```python
from build123d import *

# Parameters (mm, degrees)
SKETCH_1_W      = 62.995
SKETCH_1_H      = 25
SKETCH_1_R      = 1.4
EXTRUDE_1_DEPTH = 2.5


with BuildPart() as part:
    # 草图1 → 凸台-拉伸1 (new body, symmetric)
    with BuildSketch(Plane(origin=(0, 0, 0), x_dir=(0, 0, -1), z_dir=(1, 0, 0))):
        with Locations((31.4975, 12.5)):
            Rectangle(SKETCH_1_W, SKETCH_1_H)
        with Locations((4.995, 4.5)):
            Circle(SKETCH_1_R, mode=Mode.SUBTRACT)
        with Locations((4.995, 20.5)):
            Circle(SKETCH_1_R, mode=Mode.SUBTRACT)
        with Locations((42.995, 12.5)):
            Circle(SKETCH_1_R, mode=Mode.SUBTRACT)
        with Locations((57.995, 12.5)):
            Circle(SKETCH_1_R, mode=Mode.SUBTRACT)
    extrude(amount=EXTRUDE_1_DEPTH, both=True)


solid = part.part
```
Read the model definition and answer for the solid it produces. Units are mm, in the model's axes. Give positions to 0.01 mm unless a question says otherwise; leave off trailing zeros. Loops run counter-clockwise (first coordinate to the right, second up) from the corner with the lowest first, then second, coordinate; pieces in that order, holes last.
Item 1: The part is cut by section C-C (x = -1). Write down the section's boundary in (y, z) (3 decimals).
Item 2: The part is cut by section D-D (y = 21.25). Write down the section's boundary in (x, z) (3 decimals), and give its area (3 significant figures).
Item 3: The part is cut by section A-A (y = 12.5). Write down the section's boundary in (x, z) (3 decimals).
Item 4: The part is cut by section B-B (y = 4.5). Write down the section's boundary in (x, z) (3 decimals), and give its area (3 significant figures).
Item 5: Find the intervals of material crossed by line 1 along Z through (x, y) = (-1, 13) (3 decimals); line 2 along Z through (x, y) = (-1.45, 12.75) (1 decimal); line 3 along Y through (x, z) = (0.1, -58.5), in increasing order.
Item 6: This flat-tipped pin is pushed along its axis until it touches: pin 1 Ø3 at (x, y) = (1, 4) entering from +Z. Where does it stop, or does it pass through?
Item 7: The mould has two halves that part along Y. Classify faces 1 (the flat face through (-2.5, 13, -31)), 2 (the flat face through (0, 25, -31)), 3 (the cylindrical face through (-0.035, 19.133, -4.692)): released by +Y, released by -Y, zero draft, split by the parting line, or undercut.
Taken from the geometry:
1. outline: (0, -62.995) - (25, -62.995) - (25, 0) - (0, 0) - close; hole circle Ø2.8 at (4.5, -4.995); hole circle Ø2.8 at (12.5, -57.995); hole circle Ø2.8 at (12.5, -42.995); hole circle Ø2.8 at (20.5, -4.995)
2. outline: (-2.5, -62.995) - (2.5, -62.995) - (2.5, -6.177) - (-2.5, -6.177) - close; (-2.5, -3.813) - (2.5, -3.813) - (2.5, 0) - (-2.5, 0) - close
2. area: 303 mm2
3. outline: (-2.5, -62.995) - (2.5, -62.995) - (2.5, -59.395) - (-2.5, -59.395) - close; (-2.5, -56.595) - (2.5, -56.595) - (2.5, -44.395) - (-2.5, -44.395) - close; (-2.5, -41.595) - (2.5, -41.595) - (2.5, 0) - (-2.5, 0) - close
4. outline: (-2.5, -62.995) - (2.5, -62.995) - (2.5, -6.395) - (-2.5, -6.395) - close; (-2.5, -3.595) - (2.5, -3.595) - (2.5, 0) - (-2.5, 0) - close
4. area: 301 mm2
5. line 1: z = -62.995 to -59.303, -56.687 to -44.303, -41.687 to 0
5. line 2: z = -63 to -59.4, -56.6 to -44.4, -41.6 to 0
5. line 3: y = 0 to 11.19, 13.81 to 25
6. pin 1: stops at z = 0
7. face 1: zero draft
7. face 2: released by +Y
7. face 3: undercut
